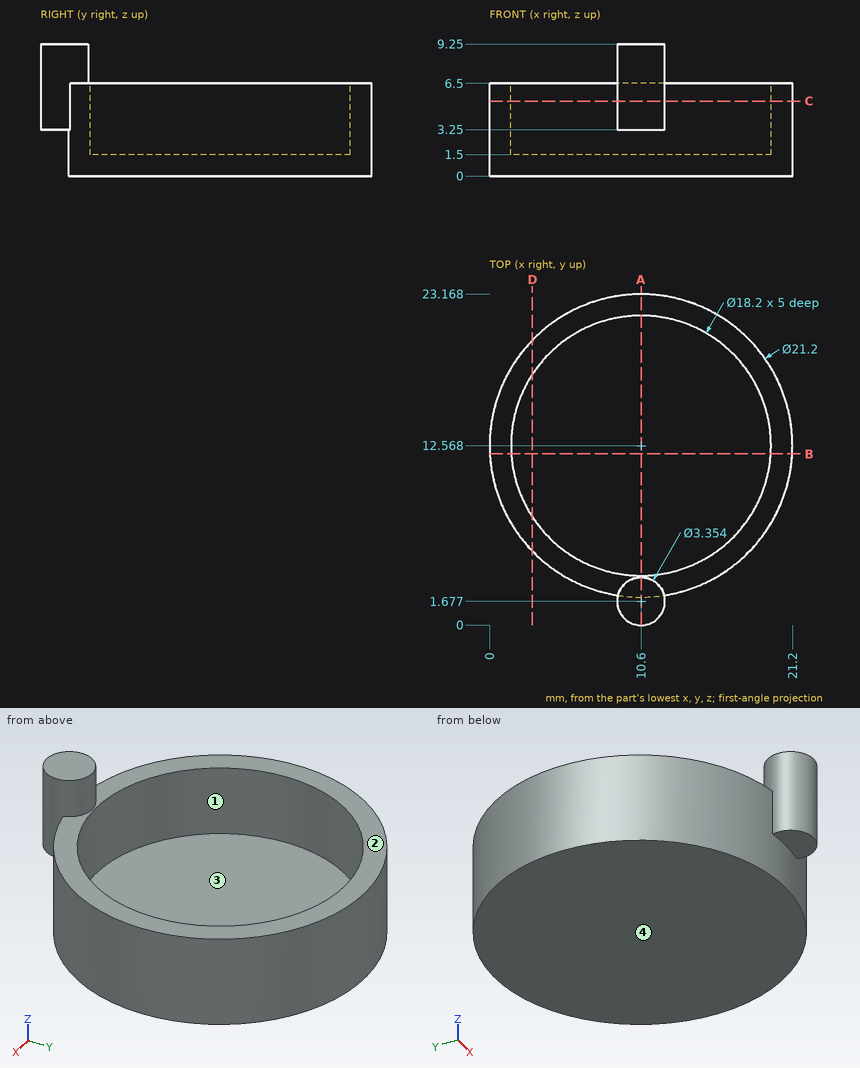
Source: three-view drawing plus pictorial views. Frame: mm from the lowest corner of the part. A direction names the side the tool comes from. Round coordinates to 2 decimals unless told otherwise and drop trailing zeros. Order: outer loops, then holes, each group sorted by start corner. A loop starts at its lowest first (then second) coordinate and runs counter-clockwise, first axis right, second up. Notation, with made-up numbers: M 60.25,85 L 95.25,85 A34 ccw 95.25,123 Z; hole C -3.75,-4.5 d10. An arc over 180 degrees is marked long. One line per item, written item: value.
(1) Line query: probe 1 along Y at (x, z) = (10.6, 4.15); probe 2 along Y at (x, z) = (10.6, 2.6); probe 3 along Z at (x, y) = (4.5, 8.75). Output: solid intervals per line, ascending. Write a range as [from, to].
Result sheet:
probe 1: [0, 3.47], [21.67, 23.17]
probe 2: [1.97, 3.47], [21.67, 23.17]
probe 3: [0, 1.5]
(2) Cut plane C-C (z = 5.25). Return the cut outline in (x, y) (1 decimal).
Result sheet:
outline: M 9,2.1 A1.7 ccw long 12.2,2.1 A10.6 ccw long Z; hole C 10.6,12.6 d18.2
(3) Cut plane B-B (y = 12). Return the cut outline in (x, z) (1 decimal).
Result sheet:
outline: M 0,0 L 21.2,0 L 21.2,6.5 L 19.7,6.5 L 19.7,1.5 L 1.5,1.5 L 1.5,6.5 L 0,6.5 Z
(4) Pull-direction query (Y, two-part tool) for the marked faces 1 and 2; classes: pulls with the +Y half, pulls with the -Y half, needs draft (parallel to the pull), parting line crosses it, or undercut.
Result sheet:
face 1: undercut
face 2: needs draft
(5) Cut plane D-D (x = 3). Return the cut outline in (y, z).
Result sheet:
outline: M 5.18,0 L 19.96,0 L 19.96,6.5 L 17.57,6.5 L 17.57,1.5 L 7.56,1.5 L 7.56,6.5 L 5.18,6.5 Z
(6) Reachability of the marked faces 3 and 4 from +Z, -Z, +X, -X, +Y, -Y: full face, straight path, thin tool, end or side. Return the list, or none.
Result sheet:
face 3: +Z
face 4: -Z, +X, -X, +Y, -Y
(7) Pin query (flat end, axial travel): P1, Ø3, axis at y = 5.5, z = 5.5, coming from the +X side; P2, Ø1, axis at x = 2.5, z = 2.5, coming from the -Y side; P3, Ø1.5, axis at y = 15.5, z = 3, coming from the +X side. Return the tip coordinate at first contact, or that it passes through.
Result sheet:
P1: x = 19.62
P2: y = 5.18
P3: x = 20.97
(8) Cut plane A-A (x = 10.6). Return the cut outline in (y, z).
Result sheet:
outline: M 0,3.25 L 1.97,3.25 L 1.97,0 L 23.17,0 L 23.17,6.5 L 21.67,6.5 L 21.67,1.5 L 3.47,1.5 L 3.47,6.5 L 3.35,6.5 L 3.35,9.25 L 0,9.25 Z
